```python
from build123d import *

# Parameters (mm, degrees)
F1_DEPTH = 38.1
F3_DEPTH = 12.7
F5_DEPTH = 12.7
F7_DEPTH = 25.4
F9_DEPTH = 50.8


with BuildPart() as f1:
    # F0 (on Right) → F1 (new body)
    with BuildSketch(Plane.YZ):
        Polygon((0, 0), (0, 31.75), (-63.5, 32.545739), (-63.5, 0), align=None)
    extrude(amount=F1_DEPTH)

    # F2 (on face) → F3 (cut)
    with BuildSketch(Plane(origin=(0, 0, 0), x_dir=(0, -1, 0), z_dir=(-1, 0, 0))):
        Polygon((63.5, 32.545739), (19.05, 31.988722), (38.1, 0), (63.5, 0), align=None)
    extrude(amount=-F3_DEPTH, mode=Mode.SUBTRACT)

    # F4 (on face) → F5 (join)
    with BuildSketch(Plane.YZ.offset(38.1)):
        Polygon((0, 31.75), (-19.05, 31.988722), (-38.1, 0), (0, 0), align=None)
    extrude(amount=F5_DEPTH)

    # F6 (on face) → F7 (cut)
    with BuildSketch(Plane(origin=(12.7, 0, 0), x_dir=(0, -1, 0), z_dir=(-1, 0, 0))):
        Polygon((63.5, 32.545739), (50.8, 32.386591), (63.5, 0), align=None)
    extrude(amount=F7_DEPTH, mode=Mode.SUBTRACT)

    # F8 (on face) → F9 (cut)
    with BuildSketch(Plane(origin=(12.7, 0, 0), x_dir=(0, -1, 0), z_dir=(-1, 0, 0))):
        Polygon((63.5, 32.545739), (50.8, 32.386591), (63.5, 0), align=None)
    extrude(amount=-F9_DEPTH, mode=Mode.SUBTRACT)


solid = f1.part
```
Build history of the part. All positions in model axes, mm. A direction names the side the tool comes from. Round coordinates to 2 decimals unless told otherwise and drop trailing zeros. Write each loop counter-clockwise with the first axis right and the second up, starting at its lowest first coordinate (ties: lowest second). Pieces come first, ordered by that corner, then holes. Notation, with made-up numbers: (34.5, 19) - (81.5, 19) arc R23 ccw to (81.5, 29) - close; hole circle Ø8 at (30.5, 29.5). An arc over 180 degrees is marked (long way). Write each question's results on one line, items separated by ' | '. Start each with the question number.
Item 1: Saw through at A-A (z = 26.5). Write the cut outline in (x, y).
Item 2: Drop flat-ended pins along their axis: P1, Ø3, axis at y = -41, z = 7.5, coming from the +X side; P2, Ø1, axis at y = -35.5, z = 6.5, coming from the -X side; P3, Ø1, axis at x = 6, y = -38.5, coming from the +Z side. Give the stop position or say it passes through.
Item 3: Saw through at B-B (y = -25). Write the cut outline in (x, z).
Item 4: Saw through at C-C (x = 21). Write the cut outline in (y, z), and give its area (3 significant figures).
Item 5: Wall check: L1, parallel to X at y = -55, z = 17.5; L2, parallel to Y at x = 37, z = 30.5; L3, parallel to Z at x = 11.5, y = -27. Give the ranges that are in metal, low to high. Write a range as [from, to].
Item 6: Which spindle directions (+Z, -Z, +X, -X, +Y, -Y) get a long thin tool onto all of the face, cutting with end or side? Do faces 1 (the face through (25, -25, 0)), 2 (the face through (38.1, -42, 16)), 3 (the face through (6.26, -28.44, 16.22)). Say none if no direction does.
Item 7: Saw through at D-D (x = 9.5). Write the cut outline in (y, z), and give its area (3 significant figures).
Results are:
1) outline: (0, -22.32) - (12.7, -22.32) - (12.7, -53.11) - (38.1, -53.11) - (38.1, -22.32) - (50.8, -22.32) - (50.8, 0) - (0, 0) - close
2) P1: stops at x = 38.1 | P2: stops at x = 12.7 | P3: stops at z = 0.17
3) outline: (0, 0) - (50.8, 0) - (50.8, 22) - (38.1, 22) - (38.1, 32.06) - (12.7, 32.06) - (12.7, 22) - (0, 22) - close
4) outline: (-63.5, 0) - (0, 0) - (0, 31.75) - (-50.8, 32.39) - close | area: 1,830 mm²
5) L1: x = [12.7, 38.1] | L2: y = [-51.54, 0] | L3: z = [0, 18.64]
6) face 1: -Z, +X, -X, +Y, -Y | face 2: +Z, +X, -Y | face 3: +Z, -X, -Y
7) outline: (-38.1, 0) - (0, 0) - (0, 31.75) - (-19.05, 31.99) - close | area: 912 mm²
